Design review of the part built by this model. Coordinates are the model's own, in mm. Give positions to 0.01 mm unless a question says otherwise; leave off trailing zeros. Order: outer loops, then holes, each group sorted by start corner. A loop starts at its lowest first (then second) coordinate and runs counter-clockwise, first axis right, second up. Notation, with made-up numbers: M 55,-10 L 83,-10 A24 cw 83,0 Z; hole C 15.25,67 d10. An arc over 180 degrees is marked long. Answer as a JSON object with one key per item and string values.
from build123d import *

# Parameters (mm, degrees)
SKETCH1_W           = 455
SKETCH1_H           = 3
BOSS_EXTRUDE1_DEPTH = 50
SKETCH2_W           = 60
SKETCH2_H           = 20
CUT_EXTRUDE1_DEPTH  = 55
CUT_EXTRUDE2_DEPTH  = 233.934540161


with BuildPart() as part:
    # Sketch1 → Boss-Extrude1 (new body)
    with BuildSketch(Plane(origin=(0, 0, 0), x_dir=(1, 0, 0), z_dir=(0, 1, 0))):
        Rectangle(SKETCH1_W, SKETCH1_H)
    extrude(amount=BOSS_EXTRUDE1_DEPTH)

    # Sketch2 → Cut-Extrude1 (cut)
    with BuildSketch(Plane.XY.offset(1.5)):
        with Locations((182.5, 10)):
            Rectangle(SKETCH2_W, SKETCH2_H)
    extrude(amount=-CUT_EXTRUDE1_DEPTH, mode=Mode.SUBTRACT)

    # Sketch3 → Cut-Extrude2 (cut, through all)
    with BuildSketch(Plane(origin=(0, 50, 0), x_dir=(1, 0, 0), z_dir=(0, 1, 0))):
        Polygon((-227.5, 1.5), (-227.5, -1.5), (-224.5, 1.5), align=None)
        Polygon((227.5, 1.5), (227.5, -1.5), (224.5, 1.5), align=None)
    extrude(amount=-CUT_EXTRUDE2_DEPTH, mode=Mode.SUBTRACT)


solid = part.part
(1) Insertion check: pin 1 (1 mm diameter, centred on y = 25.5, z = -1, fed in from -X); pin 2 (0.9 mm diameter, centred on y = 6, z = -0.5, fed in from -X); pin 3 (0.9 mm diameter, centred on x = 188.5, z = 0.5, fed in from -Y). Each pin has a flat end and moves straight along its axis. Give the tip position at first contact, or say it passes through.
Checked values:
{"pin 1": "stops at x = -225.5", "pin 2": "stops at x = -225.95", "pin 3": "stops at y = 20"}
(2) To check wall thickness, follow L1, parallel to X at y = 12, z = 0.95; L2, parallel to X at y = 6, z = -0.8; L3, parallel to Y at x = 162, z = -0.5. State the ranges of each line that lie inside material, in increasing order. Write a range as from..to.
Checked values:
{"L1": "x = -226.95..152.5, 212.5..226.95", "L2": "x = -225.2..152.5, 212.5..225.2", "L3": "y = 20..50"}
(3) We need section A-A (y = 11). Write out the cut boundary in (x, z).
Checked values:
{"outline": "M -227.5,1.5 L -224.5,-1.5 L 152.5,-1.5 L 152.5,1.5 Z; M 212.5,-1.5 L 224.5,-1.5 L 227.5,1.5 L 212.5,1.5 Z"}
(4) We need section B-B (z = -0.4). Write out the cut boundary in (x, y).
Checked values:
{"outline": "M -225.6,0 L 152.5,0 L 152.5,20 L 212.5,20 L 212.5,0 L 225.6,0 L 225.6,50 L -225.6,50 Z"}
(5) We need section C-C (x = 163). Write out the cut boundary in (y, z).
Checked values:
{"outline": "M 20,-1.5 L 50,-1.5 L 50,1.5 L 20,1.5 Z"}
